The model under review builds one solid part; all positions refer to its coordinate system, in mm. Give positions to 0.01 mm unless a question says otherwise; leave off trailing zeros. Order: outer loops, then holes, each group sorted by start corner. A loop starts at its lowest first (then second) coordinate and runs counter-clockwise, first axis right, second up.
```python
from build123d import *

# Parameters (mm, degrees)
SCALE1_SCALE = 1.9329
SCALE2_SCALE = 1.5


with BuildPart() as part:
    # Sketch3 → Revolve1 (revolve)
    with BuildSketch(Plane.XY, mode=Mode.PRIVATE) as revolve1_sk:
        with BuildLine():
            Line((-7.5, 36), (-7.5, 41))
            Line((-7.5, 41), (7.5, 41))
            Line((7.5, 41), (7.5, 36))
            Line((7.5, 36), (6.873863542, 36))
            ThreePointArc((6.873863542, 36), (0, 40.5), (-6.873863542, 36))
            Line((-6.873863542, 36), (-7.5, 36))
        make_face()
    revolve(revolve1_sk.sketch.rotate(Axis((0, 0, 0), (1, 0, 0)), 90), axis=Axis((0, 0, 0), (1, 0, 0)))


with BuildPart() as part_1:
    # Scale1: scaled about (0, 0, 0)
    add(part.part.scale(SCALE1_SCALE))


with BuildPart() as part_2:
    # Scale2: scaled about (0, 0, 0)
    add(part_1.part.scale(SCALE2_SCALE))


solid = part_2.part
```
Item 1: For line 1 (Y direction, x = -20.45, z = 0); line 2 (Z direction, x = -14, y = -76.5); line 3 (Z direction, x = 2.5, y = 65), list the stretches that pass through material, from the lowest coordinate up.
Values found:
line 1: y = -118.87 to -104.38, 104.38 to 118.87
line 2: z = -90.99 to -82.24, 82.24 to 90.99
line 3: z = -99.53 to -97.62, 97.62 to 99.53
Item 2: Take a section at A-A (z = 0). Give the boundary of the cut face in (x, y), and give its area (3 significant figures).
Values found:
outline: (-21.75, -118.87) - (21.75, -118.87) - (21.75, -104.38) - (19.93, -104.38) arc R21.75 cw to (-19.93, -104.38) - (-21.75, -104.38) - close; (-21.75, 104.38) - (-19.93, 104.38) arc R21.75 cw to (19.93, 104.38) - (21.75, 104.38) - (21.75, 118.87) - (-21.75, 118.87) - close
area: 511 mm2
Item 3: Draft analysis for pull direction Z (two halves, no side actions). For faces 1 (the cylindrical face through (0.304, 116.047, -25.769)), 2 (the cylindrical face through (-20.85, -31.352, 99.557)), 3 (the flat face through (21.745, 105, -1)), state which applies: released by +Z, released by -Z, zero draft, split by the parting line, or undercut.
Values found:
face 1: split by the parting line
face 2: undercut
face 3: zero draft
Item 4: Take a section at C-C (x = -10). Give the boundary of the cut face in (y, z), and give its area (3 significant figures).
Values found:
outline: circle Ø237.75 at (0, 0); hole circle Ø229.98 at (0, 0)
area: 2,850 mm2
Item 5: Clearance check with flat-ended pins moving along their axes: pin 1 Ø1 at (x, z) = (-17.5, 63.5) entering from -Y; pin 2 Ø12 at (x, y) = (-14.5, -54) entering from +Z; pin 3 Ø10 at (x, z) = (-8, -63.5) entering from +Y. State where each tip first meets the part, or that it passes through.
Values found:
pin 1: stops at y = -100.81
pin 2: stops at z = 108.75
pin 3: stops at y = 103.48
Item 6: Take a section at D-D (x = 5.5). Give the boundary of the cut face in (y, z), and give its area (3 significant figures).
Values found:
outline: circle Ø237.75 at (0, 0); hole circle Ø233.43 at (0, 0)
area: 1,600 mm2
